Here's how the part is built. I have some questions about the finished solid (model axes, mm). Face numbers are marked on the shaded views. A direction names the side the tool comes from. Round coordinates to 2 decimals unless told otherwise and drop trailing zeros. Loops run counter-clockwise (first coordinate to the right, second up) from the corner with the lowest first, then second, coordinate; pieces in that order, holes last. Notation, with made-up numbers: M 32.25,13 L 65.25,13 A24 cw 65.25,43 Z; hole C 47.25,-19 d4. An arc over 180 degrees is marked long. Write each question's results on one line, items separated by ' | '. Start each with the question number.
```python
from build123d import *

# Parameters (mm, degrees)
SKETCH1_W           = 170
SKETCH1_H           = 140
BOSS_EXTRUDE1_DEPTH = 3
SKETCH3_W           = 170
SKETCH3_H           = 140
SKETCH3_W_2         = 164
SKETCH3_H_2         = 134
BOSS_EXTRUDE2_DEPTH = 120
CUT_EXTRUDE1_REACH  = 206.827
SKETCH4_W           = 130
SKETCH4_H           = 10.3
SKETCH5_W           = 75
SKETCH5_H           = 52
CUT_EXTRUDE2_DEPTH  = 40
BOSS_EXTRUDE3_DEPTH = 49
CUT_EXTRUDE3_REACH  = 206.827
SKETCH8_R           = 2.25
CUT_EXTRUDE4_REACH  = 223.199
SKETCH9_W           = 75
SKETCH9_H           = 49
FILLET1_R           = 3
CHAMFER1_SIZE       = 1.5
CHAMFER1_SIZE2      = 2.14222201
FILLET2_R           = 10


with BuildPart() as part:
    # Sketch1 → Boss-Extrude1 (new body)
    with BuildSketch(Plane(origin=(0, 0, 0), x_dir=(1, 0, 0), z_dir=(0, 1, 0))):
        Rectangle(SKETCH1_W, SKETCH1_H)
    extrude(amount=BOSS_EXTRUDE1_DEPTH)

    # Sketch3 → Boss-Extrude2 (add)
    with BuildSketch(Plane(origin=(0, 3, 0), x_dir=(1, 0, 0), z_dir=(0, 1, 0))):
        Rectangle(SKETCH3_W, SKETCH3_H)
        Rectangle(SKETCH3_W_2, SKETCH3_H_2, mode=Mode.SUBTRACT)
    extrude(amount=BOSS_EXTRUDE2_DEPTH)

    # Sketch4 → Cut-Extrude1 (cut, up to next)
    with BuildSketch(Plane.XY.offset(70), mode=Mode.PRIVATE) as cut_extrude1_sk1:
        with Locations((17, 117.85)):
            Rectangle(SKETCH4_W, SKETCH4_H)
    cut_extrude1_tool1 = extrude(cut_extrude1_sk1.sketch, amount=-CUT_EXTRUDE1_REACH, mode=Mode.PRIVATE) & part.part
    add(cut_extrude1_tool1.solids().sort_by_distance((17, 117.85, 70))[0], mode=Mode.SUBTRACT)

    # Sketch5 → Cut-Extrude2 (cut)
    with BuildSketch(Plane.ZY.offset(85)):
        with Locations((32.5, 26)):
            Rectangle(SKETCH5_W, SKETCH5_H)
    extrude(amount=-CUT_EXTRUDE2_DEPTH, mode=Mode.SUBTRACT)

    # Sketch6 → Boss-Extrude3 (add)
    with BuildSketch(Plane(origin=(0, 3, 0), x_dir=(1, 0, 0), z_dir=(0, 1, 0))):
        Polygon((-45, 5), (-45, -67), (-42, -67), (-42, 8), (-82, 8), (-82, 5), align=None)
    extrude(amount=BOSS_EXTRUDE3_DEPTH)

    # Sketch8 → Cut-Extrude3 (cut, up to next)
    with BuildSketch(Plane.XY.offset(70), mode=Mode.PRIVATE) as cut_extrude3_sk1:
        with Locations((67, 92.7)):
            Circle(SKETCH8_R)
    cut_extrude3_tool1 = extrude(cut_extrude3_sk1.sketch, amount=-CUT_EXTRUDE3_REACH, mode=Mode.PRIVATE) & part.part
    # Sketch8 → Cut-Extrude3 (cut, up to next)
    with BuildSketch(Plane.XY.offset(70), mode=Mode.PRIVATE) as cut_extrude3_sk2:
        with Locations((-33, 92.7)):
            Circle(SKETCH8_R)
    cut_extrude3_tool2 = extrude(cut_extrude3_sk2.sketch, amount=-CUT_EXTRUDE3_REACH, mode=Mode.PRIVATE) & part.part
    add(cut_extrude3_tool1.solids().sort_by_distance((67, 92.7, 70))[0], mode=Mode.SUBTRACT)
    add(cut_extrude3_tool2.solids().sort_by_distance((-33, 92.7, 70))[0], mode=Mode.SUBTRACT)

    # Sketch9 → Cut-Extrude4 (cut, up to next)
    with BuildSketch(Plane(origin=(85, 0, 0), x_dir=(0, 0, -1), z_dir=(1, 0, 0)), mode=Mode.PRIVATE) as cut_extrude4_sk1:
        with Locations((-29.5, 27.5)):
            Rectangle(SKETCH9_W, SKETCH9_H)
    cut_extrude4_tool1 = extrude(cut_extrude4_sk1.sketch, amount=-CUT_EXTRUDE4_REACH, mode=Mode.PRIVATE) & part.part
    add(cut_extrude4_tool1.solids().sort_by_distance((85, 27.5, 29.5))[0], mode=Mode.SUBTRACT)

    # Fillet1
    fillet1_edges = [part.edges().sort_by_distance(p)[0] for p in [
        (-45, 26, -5),
        (-45, 26, 70),
        (-85, 26, -5),
        (-42, 27.5, -8),
        (85, 61.5, 70),
        (-85, 87.5, 70),
        (-85, 61.5, -70),
        (85, 61.5, -70),
    ]]
    fillet(fillet1_edges, radius=FILLET1_R - 0.0001)  # a hair under: the kernel refuses the full size

    # Chamfer1
    chamfer1_edges = [part.edges().sort_by_distance(p)[0] for p in [
        (-45, 0, 32.5),
        (20, 0, 70),
        (-65, 0, -5),
        (-85, 0, -37.5),
        (0, 0, -70),
        (85, 0, 0),
        (-84.121349633, 0, -69.121349633),
        (84.121349633, 0, 69.121349633),
        (84.121349633, 0, -69.121349633),
        (-84.121349633, 0, -5.878650367),
        (-44.121349633, 0, 69.121349633),
        (-45.878650367, 0, -4.121349633),
    ]]
    chamfer1_side = [part.faces().sort_by_distance(p)[0] for p in [
        (9.378358702, 0, -4.68911711),
    ]]
    chamfer(chamfer1_edges, length=CHAMFER1_SIZE, length2=CHAMFER1_SIZE2, reference=chamfer1_side[0])

    # Fillet2
    fillet2_edges = [part.edges().sort_by_distance(p)[0] for p in [
        (83.5, 52, 67),
        (83.5, 52, -8),
        (83.5, 3, -8),
    ]]
    fillet(fillet2_edges, radius=FILLET2_R)


solid = part.part
```
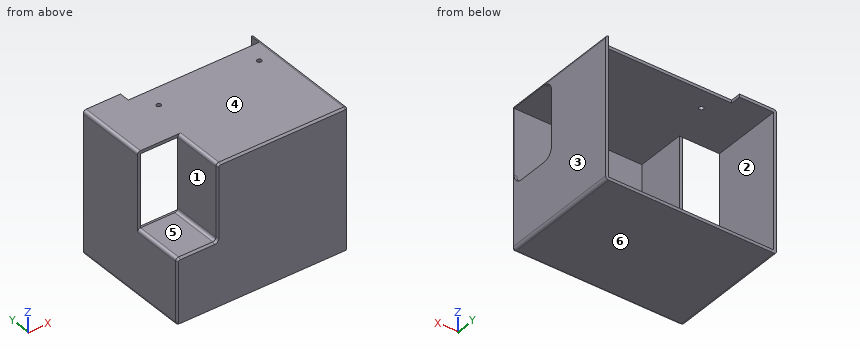
1. I want a section at D-D on y = 92.7. List the corners of the cut face in (x, z) for me.
2. I want a section at C-C on x = 67. List the corners of the cut face in (y, z) for me, plus the area to 3 significant figures.
3. Which directions (+Z, -Z, +X, -X, +Y, -Y) give clear straight access to the entire face, cutting with the end or side of a thin tool? Please do the marked faces 5 and 6.
4. I want a section at B-B on y = 67.5. List the corners of the cut face in (x, z) for me, plus the area to 3 significant figures.
5. For pin 1 (2.5 mm diameter, centred on y = 116, z = 69, fed in from +X); pin 2 (2.5 mm diameter, centred on x = 84, y = 27.5, fed in from +Z); pin 3 (0.9 mm diameter, centred on x = 40, z = 68, fed in from +Y), each with a flat end and sliding along its axis, tell me the tip position at first contact or that it passes through.
6. I want a section at A-A on z = 26. List the corners of the cut face in (x, y) for me.
7. I need wall thicknesses on line 1 along Z through (x, y) = (-29.5, 7.5); line 2 along Z through (x, y) = (-59, 32.5); line 3 along X through (y, z) = (29, -54). Which ranges of each line are inside material? Lowest first, please.
8. If we mould it in two halves opening along X, with no side actions, what happens to the marked faces 1, 2, 3 and 4? For each: released by +X, released by -X, zero draft, split by the parting line, or undercut.
Outcome:
1) outline: M -85,-67 A3 ccw -82,-70 L 82,-70 A3 ccw 85,-67 L 85,67 A3 ccw 82,70 L 69.25,70 L 69.25,67 L 82,67 L 82,-67 L -82,-67 L -82,67 L -35.25,67 L -35.25,70 L -82,70 A3 ccw -85,67 Z; M -30.75,67 L 64.75,67 L 64.75,70 L -30.75,70 Z
2) outline: M 0,-68.5 L 2.14,-70 L 123,-70 L 123,-67 L 3,-67 L 3,67 L 90.45,67 L 90.45,70 L 2.14,70 L 0,68.5 Z; M 94.95,67 L 112.7,67 L 112.7,70 L 94.95,70 Z | area: 1,090 mm2
3) face 5: +Z, -X, +Y, -Y | face 6: -Z, +X, -X, +Y, -Y
4) outline: M -85,-67 A3 ccw -82,-70 L 82,-70 A3 ccw 85,-67 L 85,67 A3 ccw 82,70 L -82,70 A3 ccw -85,67 Z; hole M -82,-67 L 82,-67 L 82,67 L -82,67 Z | area: 1,820 mm2
5) pin 1: x = 84.9 | pin 2: z = 69.9 | pin 3: y = 112.7
6) outline: M -85,52 L -82,52 L -82,123 L -85,123 Z; M -45,2.14 L -43.5,0 L 83.5,0 L 85,2.14 L 85,3 L -42,3 L -42,52 L -45,52 Z; M 82,52 L 85,52 L 85,123 L 82,123 Z
7) line 1: -70 to -67, 67 to 70 | line 2: -70 to -67, -8 to -5 | line 3: -85 to -82, 82 to 85
8) face 1: released by -X | face 2: undercut | face 3: released by +X | face 4: zero draft
